from build123d import *

# Parameters (mm, degrees)
SKETCH2_R           = 15.5
CUT_EXTRUDE1_DEPTH  = 2.5
SKETCH3_R           = 7.5
CUT_EXTRUDE2_DEPTH  = 4
SKETCH4_R           = 6.5
BOSS_EXTRUDE1_DEPTH = 10


with BuildPart() as part:
    # Sketch1 → Revolve1 (revolve)
    with BuildSketch(Plane.XY):
        with BuildLine():
            Line((0, 45), (0, 0))
            Line((0, 0), (-7.5, 0))
            add(Edge.make_bspline(
                [(-20.5, 45), (-20.945482832, 16.446098589), (-7.5, 0)],
                knots=[0, 0, 0, 0.557031676, 0.557031676, 0.557031676], degree=2))
            Line((-20.5, 45), (0, 45))
        make_face()
    revolve(axis=Axis((0, 45, 0), (0, -1, 0)))

    # Sketch2 → Cut-Extrude1 (cut)
    with BuildSketch(Plane(origin=(0, 45, 0), x_dir=(1, 0, 0), z_dir=(0, 1, 0))):
        with Locations(Location((0, 0, 0), (0, 0, 270))):
            Circle(SKETCH2_R)
    extrude(amount=-CUT_EXTRUDE1_DEPTH, mode=Mode.SUBTRACT)

    # Sketch3 → Cut-Extrude2 (cut)
    with BuildSketch(Plane(origin=(0, 45, 0), x_dir=(1, 0, 0), z_dir=(0, 1, 0))):
        with Locations(Location((0, 0, 0), (0, 0, 270))):
            Circle(SKETCH3_R)
    extrude(amount=-CUT_EXTRUDE2_DEPTH, mode=Mode.SUBTRACT)

    # Sketch4 → Boss-Extrude1 (add)
    with BuildSketch(Plane.XZ):
        with Locations(Location((0, 0, 0), (0, 0, 270))):
            Circle(SKETCH4_R)
    extrude(amount=BOSS_EXTRUDE1_DEPTH)

    # Sketch6 → Cut-Revolve1 (revolve, cut)
    with BuildSketch(Plane.XY):
        with BuildLine():
            Line((0, 36), (0, 0))
            Line((0, 0), (0, -10))
            Line((0, -10), (-2.5, -10))
            Line((-2.5, -10), (-2.5, 0))
            add(Edge.make_bspline(
                [(-15.275259687, 36), (-14.25878691, 21.174216867), (-10.000367015, 9.174216867), (-2.5, 0)],
                knots=[0.09093365, 0.09093365, 0.09093365, 0.09093365, 0.557031676, 0.557031676, 0.557031676, 0.557031676], degree=3))
            Line((-15.275259687, 36), (0, 36))
        make_face()
    revolve(axis=Axis((0, 36, 0), (0, -1, 0)), mode=Mode.SUBTRACT)


solid = part.part
Input: part model. Units: mm. Frame: model coordinates. A direction names the side the tool comes from. Coordinates: 2 decimals unless noted, no trailing zeros. Answer as a JSON object with one key per item and string values. Group by question number.
(1) Mould query, pull axis X, two halves, no side actions, for faces 5 (the face through (0, 41, 0)), 6 (the face through (0.33, 41.76, -7.493)), 7 (the face through (8, 45, -14)), 8 (the face through (-3.955, -4.93, 5.158)). Classes: pulls with the +X half, pulls with the -X half, needs draft (parallel to the pull), parting line crosses it, or undercut.
(2) Ray query, line 1 along X through (y, z) = (-5.5, 0); line 2 along X through (y, z) = (25, -9); line 3 along Z through (x, y) = (4, 22). Return the intervals inside material, ascending. Write a range as [from, to].
(3) Contact query for flat-ended pins moving along their axis: P1, Ø4.5, axis at x = 0, z = 0, coming from the +Y side; P2, Ø2, axis at x = -4, z = 9.5, coming from the -Y side; P3, Ø16.5, axis at x = -3.5, z = 1, coming from the +Y side; P4, Ø7.5, axis at x = 2, z = -0.5, coming from the -Y side. Output: stop coordinate, or through.
(4) Set-up query: faces 1 (the face through (0, 36, 0)), 2 (the face through (0.54, -4.93, 2.44)), 3 (the face through (4, 42.5, 7)), 4 (the face through (0, -10, -3)). Return all of +Z, -Z, +X, -X, +Y, -Y with unobstructed straight access to the full face (end or side cutting, diameter ignored); none if empty.
Result set:
{
 "1": {"face 5": "undercut", "face 6": "undercut", "face 7": "needs draft", "face 8": "parting line crosses it"},
 "2": {"line 1": "x = [-6.5, -2.5], [2.5, 6.5]", "line 2": "x = [-16.53, -10.49], [10.49, 16.53]", "line 3": "z = [-17.7, -12.53], [12.53, 17.7]"},
 "3": {"P1": "stops at y = 41", "P2": "stops at y = 2.35", "P3": "stops at y = 42.5", "P4": "stops at y = -10"},
 "4": {"face 1": "none", "face 2": "-Y", "face 3": "+Y", "face 4": "+Z, -Z, +X, -X, -Y"}
}
